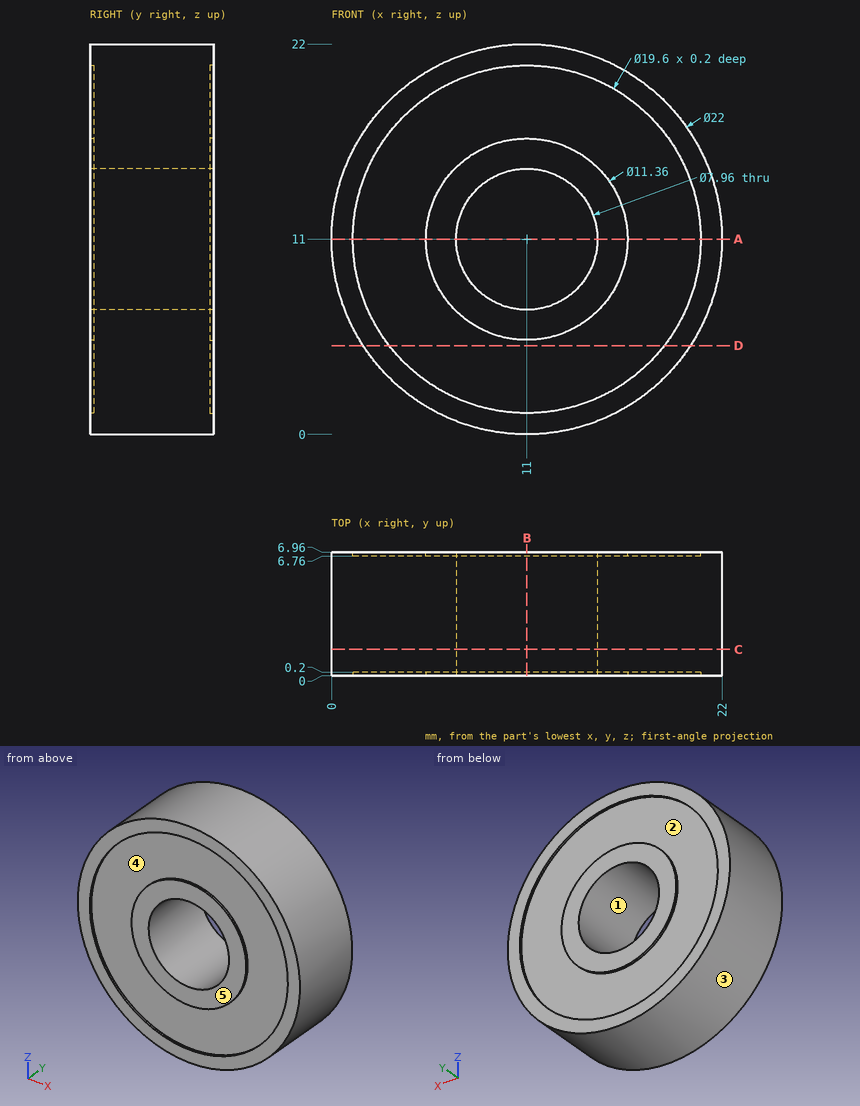
Drawing for the job (mm, zero at the part's lowest x, y, z). A direction names the side the tool comes from. Coordinates: 2 decimals unless noted, no trailing zeros. Write each loop counter-clockwise with the first axis right and the second up, starting at its lowest first coordinate (ties: lowest second). Pieces come first, ordered by that corner, then holes. Notation, with made-up numbers: (1.25, -40) - (29.25, -40) arc R28 ccw to (29.25, -21) - close; hole circle Ø3 at (-4.75, 24). An arc over 180 degrees is marked (long way). Write each question's results on one line, items separated by ' | '. Start each with the question number.
1) Cut at A-A (z = 11). Write the cut outline in (x, y), then the cut area to 3 significant figures.
2) 3-axis set-ups, long thin cutter, end or side, ignore diameter. For the marked faces 1 and 2: which of +Z, -Z, +X, -X, +Y, -Y reach the whole face in a straight line?
3) Cut at B-B (x = 11). Write the cut outline in (y, z), then the cut area to 3 significant figures.
4) Mould opens along Z. For the marked faces 3, 4 and 5 say: pulls with the +Z half, pulls with the -Z half, needs draft (parallel to the pull), parting line crosses it, or undercut.
5) Flat gauge pins, fed straight in: P1, Ø1, axis at x = 14, y = 6, coming from the -Z side; P2, Ø4, axis at x = 15, y = 4.5, coming from the +Z side; P3, Ø1.5, axis at x = 17.5, z = 17, coming from the -Y side. Where does each tip first touch, or does it go through?
6) Probe line 1 along X through (y, z) = (0.1, 11); line 2 along X through (y, z) = (4, 11); line 3 along Y through (x, z) = (10.75, 19.5). List the from-to ranges inside material, lowest first. Write a range as from..to.
7) Cut at D-D (z = 5). Write the cut outline in (x, y).
8) Cut at C-C (y = 1.5). Write the cut outline in (x, z).
Returned:
1) outline: (0, 0) - (1.2, 0) - (1.2, 0.2) - (5.32, 0.2) - (5.32, 0) - (7.02, 0) - (7.02, 6.96) - (5.32, 6.96) - (5.32, 6.76) - (1.2, 6.76) - (1.2, 6.96) - (0, 6.96) - close; (14.98, 0) - (16.68, 0) - (16.68, 0.2) - (20.8, 0.2) - (20.8, 0) - (22, 0) - (22, 6.96) - (20.8, 6.96) - (20.8, 6.76) - (16.68, 6.76) - (16.68, 6.96) - (14.98, 6.96) - close | area: 94.4 mm^2
2) face 1: +Y, -Y | face 2: +Y
3) outline: (0, 0) - (6.96, 0) - (6.96, 1.2) - (6.76, 1.2) - (6.76, 5.32) - (6.96, 5.32) - (6.96, 7.02) - (0, 7.02) - (0, 5.32) - (0.2, 5.32) - (0.2, 1.2) - (0, 1.2) - close; (0, 14.98) - (6.96, 14.98) - (6.96, 16.68) - (6.76, 16.68) - (6.76, 20.8) - (6.96, 20.8) - (6.96, 22) - (0, 22) - (0, 20.8) - (0.2, 20.8) - (0.2, 16.68) - (0, 16.68) - close | area: 94.4 mm^2
4) face 3: parting line crosses it | face 4: undercut | face 5: needs draft
5) P1: z = 0.29 | P2: z = 21.82 | P3: y = 0.2
6) line 1: 0..1.2, 5.32..7.02, 14.98..16.68, 20.8..22 | line 2: 0..7.02, 14.98..22 | line 3: 0.2..6.76
7) outline: (1.78, 0) - (3.25, 0) - (3.25, 0.2) - (18.75, 0.2) - (18.75, 0) - (20.22, 0) - (20.22, 6.96) - (18.75, 6.96) - (18.75, 6.76) - (3.25, 6.76) - (3.25, 6.96) - (1.78, 6.96) - close
8) outline: circle Ø22 at (11, 11); hole circle Ø7.96 at (11, 11)
